Autodesk Inventor part; units mm, degrees
ref_plane "YZ Plane" through (0, 0, 0) normal (1, 0, 0) x (0, 1, 0)
ref_plane "XZ Plane" through (0, 0, 0) normal (0, 1, 0) x (-1, 0, 0)
ref_plane "XY Plane" through (0, 0, 0) normal (0, 0, 1) x (1, 0, 0)
sketch "Boceto1" plane through (0, 0, 0) normal (0, 0, 1) x (1, 0, 0)
  line L0 (-83, -108.2) -> (83, -108.2)
  line L1 (83, -108.2) -> (83, 108.2)
  line L2 (83, 108.2) -> (-83, 108.2)
  line L3 (-83, 108.2) -> (-83, -108.2)
  line L4 (-83, -108.2) -> (83, 108.2) construction
  line L5 (83, -108.2) -> (-83, 108.2) construction
  point P0 (0, 0)
  dimension "d0" = 166
  dimension "d1" = 216.4
extrude "Extrusión1" add sketch "Boceto1" along normal blind 15
sketch "Boceto2" plane through (0, 0, 15) normal (0, 0, 1) x (1, 0, 0)
  line L0 (80.75, -105.95) -> (-80.75, -105.95)
  line L1 (-80.75, -105.95) -> (-80.75, 105.95)
  line L2 (80.75, 105.95) -> (-80.75, 105.95)
  line L3 (80.75, 105.95) -> (80.75, -105.95)
  line L4 (-83, 108.2) -> (83, 108.2)
  line L5 (83, 108.2) -> (83, -108.2)
  line L6 (83, -108.2) -> (-83, -108.2)
  line L7 (-83, -108.2) -> (-83, 108.2)
  point P0 (0, 0)
extrude "Extrusión2" cut sketch "Boceto2" against normal blind 12 contours L0 L1 L2 L3
sketch "Boceto3" plane through (0, 0, 3) normal (0, 0, 1) x (1, 0, 0)
  line L0 (-67.5, -92.5) -> (67.5, -92.5)
  line L1 (67.5, -92.5) -> (67.5, 92.5)
  line L2 (67.5, 92.5) -> (-67.5, 92.5)
  line L3 (-67.5, 92.5) -> (-67.5, -92.5)
  line L4 (-67.5, 87.5) -> (-72.5, 87.5)
  line L5 (-62.5, 97.5) -> (-62.5, 92.5)
  line L6 (62.5, -97.5) -> (62.5, -92.5)
  line L7 (67.5, -87.5) -> (72.5, -87.5)
  line L8 (-72.5, -87.5) -> (-67.5, -87.5)
  line L9 (-62.5, -92.5) -> (-62.5, -97.5)
  line L10 (-72.5, 87.5) -> (-77.5, 87.5)
  line L11 (-77.5, 87.5) -> (-77.5, 102.5)
  line L12 (-77.5, 102.5) -> (-62.5, 102.5)
  line L13 (-62.5, 102.5) -> (-62.5, 97.5)
  line L14 (77.5, 87.5) -> (77.5, 102.5)
  line L15 (77.5, 102.5) -> (62.5, 102.5)
  line L16 (67.5, -87.5) -> (77.5, -87.5)
  line L17 (62.5, -92.5) -> (62.5, -102.5)
  line L18 (62.5, -102.5) -> (77.5, -102.5)
  line L19 (77.5, -102.5) -> (77.5, -87.5)
  line L20 (-67.5, -87.5) -> (-77.5, -87.5)
  line L21 (-77.5, -87.5) -> (-77.5, -102.5)
  line L22 (-77.5, -102.5) -> (-62.5, -102.5)
  line L23 (-62.5, -102.5) -> (-62.5, -97.5)
  line L24 (67.5, 87.5) -> (77.5, 87.5)
  line L25 (62.5, 102.5) -> (62.5, 92.5)
  arc A0 (-62.5, -92.5) -> (-67.5, -87.5) centre (-67.5, -92.5) ccw
  arc A1 (-67.5, 87.5) -> (-62.5, 92.5) centre (-67.5, 92.5) ccw
  arc A2 (62.5, 92.5) -> (67.5, 87.5) centre (67.5, 92.5) ccw
  arc A3 (67.5, -87.5) -> (62.5, -92.5) centre (67.5, -92.5) ccw
  point P0 (0, 0)
  dimension "d12" = 135
  dimension "d13" = 185
  dimension "d56" = 5
  dimension "d57" = 15
  dimension "d58" = 15
extrude "Extrusión3" add sketch "Boceto3" along normal blind 9 contours L3 A0 L0 | L0 L9 L23 L22 L21 L20 L8 L3 | A3 L1 L0 | L0 L1 L7 L16 L19 L18 L17 L6 | L4 L10 L11 L12 L13 L5 L2 L3 | L3 L2 A1 | A2 L2 L1 | L1 L2 L25 L15 L14 L24
sketch "Boceto4" plane through (0, 0, 0) normal (0, 0, -1) x (-1, 0, 0)
  line L0 (80.75, -105.95) -> (80.75, 105.95)
  line L1 (-80.75, -105.95) -> (80.75, -105.95)
  line L2 (-80.75, 105.95) -> (-80.75, -105.95)
  line L3 (80.75, 105.95) -> (-80.75, 105.95)
  line L4 (-67.5, -92.5) -> (-67.5, 92.5)
  line L5 (67.5, 92.5) -> (67.5, -92.5)
  line L6 (-67.5, 92.5) -> (67.5, 92.5)
  line L7 (67.5, -92.5) -> (-67.5, -92.5)
  circle A0 centre (-67.5, 92.5) radius 4.75
  circle A1 centre (67.5, 92.5) radius 4.75
  circle A2 centre (67.5, -92.5) radius 4.75
  circle A3 centre (-67.5, -92.5) radius 4.75
  point P0 (0, 0)
  dimension "d24" = 9.5
  dimension "d25" = 9.5
  dimension "d26" = 9.5
  dimension "d27" = 9.5
extrude "Extrusión4" cut sketch "Boceto4" against normal blind 4.5 contours L7 A3 L4 | L4 A3 L7 | A0 L6 L4 | L4 L6 A0 | A2 L5 L7 | L7 L5 A2 | A1 L5 L6 | L6 L5 A1
sketch "Boceto7" plane through (-67.5, 92.5, 4.5) normal (0, 0, -1) x (-1, 0, 0)
  arc A0 (-0.8744, -2.2886) -> (-2.2886, -0.8744) centre (0, 0) ccw
  line L0 (0, 0) -> (4.75, 0) construction
  line L1 (-2.2886, -0.8744) -> (-3.9906, -2.5764)
  line L2 (-0.8744, -2.2886) -> (-2.5764, -3.9906)
  arc A1 (-3.9906, -2.5764) -> (-2.5764, -3.9906) centre (0, 0) ccw
  arc A2 (-132.7114, -0.8744) -> (-134.1256, -2.2886) centre (-135, 0) ccw
  line L3 (-134.1256, -2.2886) -> (-132.4236, -3.9906)
  line L4 (-132.7114, -0.8744) -> (-131.0094, -2.5764)
  arc A3 (-132.4236, -3.9906) -> (-131.0094, -2.5764) centre (-135, 0) ccw
  arc A4 (-134.1256, -182.7114) -> (-132.7114, -184.1256) centre (-135, -185) ccw
  line L5 (-132.7114, -184.1256) -> (-131.0094, -182.4236)
  line L6 (-134.1256, -182.7114) -> (-132.4236, -181.0094)
  arc A5 (-131.0094, -182.4236) -> (-132.4236, -181.0094) centre (-135, -185) ccw
  arc A6 (-2.2886, -184.1256) -> (-0.8744, -182.7114) centre (0, -185) ccw
  line L7 (-0.8744, -182.7114) -> (-2.5764, -181.0094)
  line L8 (-2.2886, -184.1256) -> (-3.9906, -182.4236)
  arc A7 (-2.5764, -181.0094) -> (-3.9906, -182.4236) centre (0, -185) ccw
  point P0 (-67.5, -92.5)
extrude "Extrusión7" cut sketch "Boceto7" against normal blind 10
sketch "Boceto8" plane through (0, 0, 3) normal (0, 0, 1) x (1, 0, 0)
  line L0 (80.75, -105.95) -> (-80.75, -105.95)
  line L1 (-62.5, -105.95) -> (-57.5, -105.95)
  line L2 (-57.5, -100.95) -> (57.5161, -100.95)
  line L3 (67.5, -87.5) -> (77.5, -87.5)
  line L4 (57.5161, -92.5) -> (57.5161, -100.95)
  line L5 (-57.5, -100.95) -> (-57.5, -92.5)
  line L6 (-67.5, -82.5) -> (-75.75, -82.5)
  line L7 (-77.5, 87.5) -> (-67.5, 87.5)
  line L8 (-62.5, 92.5) -> (-62.5, 102.5)
  line L9 (-80.75, 105.95) -> (80.75, 105.95)
  line L10 (-75.75, 82.5) -> (-67.5, 82.5)
  line L11 (-57.5, 92.5) -> (-57.5, 100.95)
  line L12 (-75.75, -82.5) -> (-75.75, 82.5)
  line L13 (-57.5, 100.95) -> (57.5161, 100.95)
  line L14 (57.5161, 100.95) -> (57.5161, 91.9319)
  line L15 (67.5, 82.5) -> (75.75, 82.5)
  line L16 (75.75, 82.5) -> (75.75, -82.5161)
  arc A0 (65.2114, -91.6256) -> (66.6256, -90.2114) centre (67.5, -92.5) ccw
  line L17 (67.5, -82.5161) -> (75.75, -82.5161)
  arc A1 (-66.6256, -90.2114) -> (-65.2114, -91.6256) centre (-67.5, -92.5) ccw
  arc A2 (-57.5, -92.5) -> (-67.5, -82.5) centre (-67.5, -92.5) ccw
  arc A3 (-65.2114, 91.6256) -> (-66.6256, 90.2114) centre (-67.5, 92.5) ccw
  arc A4 (-67.5, 82.5) -> (-57.5, 92.5) centre (-67.5, 92.5) ccw
  arc A5 (67.5, -82.5161) -> (57.5161, -92.5) centre (67.5, -92.5) ccw
  arc A6 (66.6256, 90.2114) -> (65.2114, 91.6256) centre (67.5, 92.5) ccw
  arc A7 (57.5, 92.5) -> (67.5, 82.5) centre (67.5, 92.5) ccw
  point P0 (0, 0)
extrude "Extrusión8" cut sketch "Boceto8" against normal blind 10
properties part number "TestTapa_v1"
The model under review builds one solid part; all positions refer to its coordinate system, in mm. A direction names the side the tool comes from. Give positions to 0.01 mm unless a question says otherwise; leave off trailing zeros. Write each loop counter-clockwise with the first axis right and the second up, starting at its lowest first coordinate (ties: lowest second). Pieces come first, ordered by that corner, then holes.
(1) Consider section A-A, the plane x = 18. Give the boundary of the cut face in (y, z).
(2) The part is to be moulded in two halves that separate along Y. For faces 4 (the flat face through (83, -2, 7)), 5 (the flat face through (-70, -95, 12)), say which applies: released by +Y, released by -Y, zero draft, split by the parting line, or undercut.
(3) To check wall thickness, follow L1, parallel to Y at x = 67.5, z = 3.35; L2, parallel to X at y = 92.5, z = 3.25; L3, parallel to Y at x = -67.5, z = 2.15. State the ranges of each line that lie inside material, in increasing order.
(4) Tool access review of faces 1 (the flat face through (77.5, 95, 7)), 2 (the cylindrical face through (-60.35, -85.51, 1.52)), 3 (the cylindrical face through (-66.47, -97.137, 2.218)): name each direction out of +Z, -Z, +X, -X, +Y, -Y from which nothing blocks a thin tool from reaching the whole face with its end or side.
(5) For P1, Ø8, axis at x = -67.5, y = 92.5, coming from the +Z side; P2, Ø5.5, axis at x = -67.5, y = 92.5, coming from the -Z side, all flat-tipped, find the tip position at first contact; note any pin that passes through.
(6) Consider section C-C, the plane z = 9.75. Give the number of separate pieces and of enclosed holes in the cut face, and give its area (3 significant figures).
(7) Consider section B-B, the plane y = 1.5. Give the boundary of the cut face in (x, z), and give its area (3 significant figures).
Returned:
1. outline: (-108.2, 0) - (-100.95, 0) - (-100.95, 3) - (-105.95, 3) - (-105.95, 15) - (-108.2, 15) - close; (100.95, 0) - (108.2, 0) - (108.2, 15) - (105.95, 15) - (105.95, 3) - (100.95, 3) - close
2. face 4: zero draft
2. face 5: undercut
3. L1: y = -108.2 to -105.95, -102.5 to -97.25, -87.75 to -87.5, 87.5 to 87.75, 97.25 to 102.5, 105.95 to 108.2
3. L2: x = -83 to -80.75, -77.5 to -72.25, -62.75 to -62.5, 62.5 to 62.75, 72.25 to 77.5, 80.75 to 83
3. L3: y = -108.2 to -97.25, -87.75 to -82.5, 82.5 to 87.75, 97.25 to 108.2
4. face 1: +Z
4. face 2: +Z, -Z
4. face 3: -Z
5. P1: stops at z = 12
5. P2: stops at z = 4.5
6. separate pieces: 5
6. enclosed holes: 5
6. area: 2,480 mm2
7. outline: (-83, 0) - (-75.75, 0) - (-75.75, 3) - (-80.75, 3) - (-80.75, 15) - (-83, 15) - close; (75.75, 0) - (83, 0) - (83, 15) - (80.75, 15) - (80.75, 3) - (75.75, 3) - close
7. area: 97.5 mm2
